Autodesk Fusion 360 part; units mm, degrees
sketch "Sketch1" plane through (0, 0, 0) normal (0, 1, 0) x (1, 0, 0)
  circle A0 centre (0, 0) radius 20
  circle A1 centre (0, 0) radius 10
  dimension "d1" = 40
  dimension "d2" = 20
extrude "Extrude1" add sketch "Sketch1" along normal blind 30
extrude "Extrude2" add sketch "Sketch1" along normal blind 60 contours A1
fillet "Fillet1" radius 0.1 1 edges at (-9.3233, 60, 3.6162)
The listing builds one solid part. Answer for the finished solid, in the listing's coordinates (mm). A direction names the side the tool comes from. Round coordinates to 2 decimals unless told otherwise and drop trailing zeros. Order: outer loops, then holes, each group sorted by start corner. A loop starts at its lowest first (then second) coordinate and runs counter-clockwise, first axis right, second up. Notation, with made-up numbers: M -20.5,-7.5 L 28.5,-7.5 A29 cw 28.5,31.5 Z; hole C 58,56.5 d11. An arc over 180 degrees is marked long. Answer in a Markdown table with one row per item. Add a question column.
1) The part is cut by section B-B on x = 0. Determine the outline of the cut face in (y, z), plus the area to 3 significant figures.
2) Which of the six approach directions +Z, -Z, +X, -X, +Y, -Y give full straight-line access (tool end or side, diameter ignored) to faces 1 (the face through (-5, 30, -9)), 2 (the face through (0, 0, 0))?
3) The part is cut by section D-D on z = 16. Determine the outline of the cut face in (x, y).
4) The part is cut by section C-C on y = 41.5. Determine the outline of the cut face in (x, z), plus the area to 3 significant figures.
5) Flat-ended cylindrical pins translate along their axes: pin 1 Ø8 at (x, y) = (-7, 52) entering from +Z; pin 2 Ø8 at (y, z) = (14.5, -15) entering from +X; pin 3 Ø8 at (y, z) = (51.5, -10) entering from -X. Find the tip coordinate at first contact, or state that the pin passes through.
6) Consider line 1 along Y through (x, z) = (2, -17.5); line 2 along Z through (x, y) = (-7, 54); line 3 along X through (y, z) = (52, 4.5). Determine where each line is inside the solid, lowest interval first. Write a range as from..to.
7) The part is cut by section A-A on z = 0. Determine the outline of the cut face in (x, y), plus the area to 3 significant figures.
Findings below:
| question | item | result |
|---|---|---|
| 1 | outline | M 0,-20 L 30,-20 L 30,-10 L 59.9,-10 A0.1 ccw 60,-9.9 L 60,9.9 A0.1 ccw 59.9,10 L 30,10 L 30,20 L 0,20 Z |
| 1 | area | 1,800 mm² |
| 2 | face 1 | +Y |
| 2 | face 2 | +Z, -Z, +X, -X, -Y |
| 3 | outline | M -12,0 L 12,0 L 12,30 L -12,30 Z |
| 4 | outline | C 0,0 d20 |
| 4 | area | 314 mm² |
| 5 | pin 1 | stops at z = 9.54 |
| 5 | pin 2 | stops at x = 16.7 |
| 5 | pin 3 | stops at x = -8 |
| 6 | line 1 | y = 0..30 |
| 6 | line 2 | z = -7.14..7.14 |
| 6 | line 3 | x = -8.93..8.93 |
| 7 | outline | M -20,0 L 20,0 L 20,30 L 10,30 L 10,59.9 A0.1 ccw 9.9,60 L -9.9,60 A0.1 ccw -10,59.9 L -10,30 L -20,30 Z |
| 7 | area | 1,800 mm² |
